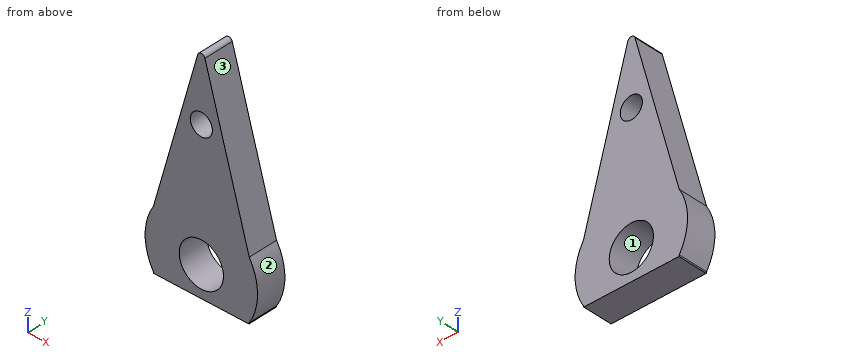
```python
from build123d import *

# Parameters (mm, degrees)
SKETCH1_R           = 3.81
BOSS_EXTRUDE1_DEPTH = 2
BOSS_EXTRUDE2_DEPTH = 2
FILLET1_R           = 0.254
SKETCH3_R           = 0.75
CUT_EXTRUDE1_DEPTH  = 2
SKETCH4_R           = 1.5
CUT_EXTRUDE2_DEPTH  = 3
CUT_EXTRUDE3_DEPTH  = 2.54


with BuildPart() as part:
    # Sketch1 → Boss-Extrude1 (new body)
    with BuildSketch(Plane(origin=(0, 0, 0), x_dir=(1, 0, 0), z_dir=(0, 1, 0))):
        Circle(SKETCH1_R)
    extrude(amount=BOSS_EXTRUDE1_DEPTH)

    # Sketch2 → Boss-Extrude2 (add)
    with BuildSketch(Plane(origin=(0, 2, 0), x_dir=(1, 0, 0), z_dir=(0, 1, 0))):
        with BuildLine():
            Line((0, -13.5), (3.247846855, -1.991881223))
            ThreePointArc((3.247846855, -1.991881223), (0, -3.81), (-3.247846855, -1.991881223))
            Line((-3.247846855, -1.991881223), (0, -13.5))
        make_face()
        with BuildLine():
            ThreePointArc((-3.247846855, 1.991881223), (0, 3.81), (3.247846855, 1.991881223))
            Line((3.247846855, 1.991881223), (0, 13.5))
            Line((0, 13.5), (-3.247846855, 1.991881223))
        make_face()
    extrude(amount=-BOSS_EXTRUDE2_DEPTH)

    # Fillet1
    fillet1_edges = [part.edges().sort_by_distance(p)[0] for p in [
        (0, 1, -13.5),
        (0, 1, 13.5),
    ]]
    fillet(fillet1_edges, radius=FILLET1_R)

    # Sketch3 → Cut-Extrude1 (cut)
    with BuildSketch(Plane(origin=(0, 2, 0), x_dir=(1, 0, 0), z_dir=(0, 1, 0))):
        with Locations((0, 8.5)):
            Circle(SKETCH3_R)
        with Locations((0, -8.5)):
            Circle(SKETCH3_R)
    extrude(amount=-CUT_EXTRUDE1_DEPTH, mode=Mode.SUBTRACT)

    # Sketch4 → Cut-Extrude2 (cut, through all)
    with BuildSketch(Plane.XZ):
        Circle(SKETCH4_R)
    extrude(amount=-CUT_EXTRUDE2_DEPTH, mode=Mode.SUBTRACT)

    # Sketch5 → Cut-Extrude3 (cut)
    with BuildSketch(Plane(origin=(0, 0, 0), x_dir=(1, 0, 0), z_dir=(0, 1, 0))):
        Polygon((5.430650193, 2.075218265), (-5.917689048, 2.075218265), (-5.917689048, 14.831745587), (0, 14.831745587), (5.430650193, 14.831745587), align=None)
    extrude(amount=CUT_EXTRUDE3_DEPTH, mode=Mode.SUBTRACT)


solid = part.part
```
Source: CAD feature listing. Evaluate the final solid. Frame: model axes, mm. Face numbers are marked on the shaded views. Round coordinates to 2 decimals unless told otherwise and drop trailing zeros. Loops run counter-clockwise (first coordinate to the right, second up) from the corner with the lowest first, then second, coordinate; pieces in that order, holes last.
1. Ray query, L1, parallel to Z at x = 0, y = 1.25; L2, parallel to X at y = 1.8, z = 8.5; L3, parallel to X at y = 1.9, z = 11. Return the intervals inside material, ascending.
2. Section query A-A on y = 0.4. Output: boundary loops of the cut face in (x, z), and give its area (3 significant figures).
3. Contact query for flat-ended pins moving along their axis: pin 1 (1.4 mm diameter, centred on x = 0, z = 8.5, fed in from -Y); pin 2 (1 mm diameter, centred on y = 1.5, z = 6.5, fed in from +X). Output: stop coordinate, or through.
4. Section query B-B on x = 1.25. Output: boundary loops of the cut face in (y, z), and give its area (3 significant figures).
5. Section query C-C on z = 0. Output: boundary loops of the cut face in (x, y).
6. Mould query, pull axis Z, two halves, no side actions, for the marked faces 1, 2 and 3. Classes: released by +Z, released by -Z, zero draft, split by the parting line, or undercut.
7. Section query D-D on x = 0. Output: boundary loops of the cut face in (y, z), and give its area (3 significant figures).
Answers below:
1. L1: z = -2.08 to -1.5, 1.5 to 7.75, 9.25 to 12.82
1. L2: x = -1.41 to -0.75, 0.75 to 1.41
1. L3: x = -0.71 to 0.71
2. outline: (-3.25, -1.99) - (-3.22, -2.08) - (3.22, -2.08) - (3.25, -1.99) arc R3.81 ccw to (3.25, 1.99) - (0.24, 12.63) arc R0.25 ccw to (-0.24, 12.63) - (-3.25, 1.99) arc R3.81 ccw to start; hole circle Ø3 at (0, 0); hole circle Ø1.5 at (0, 8.5)
2. area: 57.8 mm2
3. pin 1: passes through
3. pin 2: stops at x = 2.12
4. outline: (0, -2.08) - (2, -2.08) - (2, -0.83) - (0, -0.83) - close; (0, 0.83) - (2, 0.83) - (2, 9.07) - (0, 9.07) - close
4. area: 19.0 mm2
5. outline: (-3.81, 0) - (-1.5, 0) - (-1.5, 2) - (-3.81, 2) - close; (1.5, 0) - (3.81, 0) - (3.81, 2) - (1.5, 2) - close
6. face 1: undercut
6. face 2: split by the parting line
6. face 3: released by +Z
7. outline: (0, -2.08) - (2, -2.08) - (2, -1.5) - (0, -1.5) - close; (0, 1.5) - (2, 1.5) - (2, 7.75) - (0, 7.75) - close; (0, 9.25) - (2, 9.25) - (2, 12.82) - (0, 12.82) - close
7. area: 20.8 mm2
